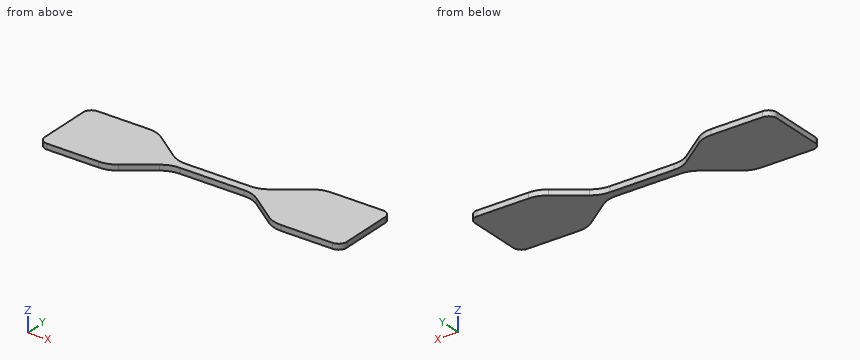
Autodesk Inventor part; units mm, degrees
ref_plane "YZ Plane" through (0, 0, 0) normal (1, 0, 0) x (0, 1, 0)
ref_plane "XZ Plane" through (0, 0, 0) normal (0, 1, 0) x (-1, 0, 0)
ref_plane "XY Plane" through (0, 0, 0) normal (0, 0, 1) x (1, 0, 0)
sketch "Sketch1" plane through (0, 0, 0) normal (0, 0, 1) x (1, 0, 0)
  line L0 (0, 0) -> (25, 0)
  line L1 (25, 25) -> (0, 25)
  line L2 (0, 25) -> (0, 0)
  line L3 (40, 14) -> (70, 14)
  line L4 (70, 11) -> (40, 11)
  line L5 (85, 0) -> (110, 0)
  line L6 (110, 0) -> (110, 25)
  line L7 (110, 25) -> (85, 25)
  line L8 (25, 25) -> (40, 14)
  line L9 (25, 0) -> (40, 11)
  line L10 (70, 14) -> (85, 25)
  line L11 (70, 11) -> (85, 0)
  point P0 (45, 12.5)
  point P1 (25, 12.5)
  dimension "d0" = 25
  dimension "d1" = 25
  dimension "d5" = 25
  dimension "d6" = 110
  dimension "d12" = 3
  dimension "d13" = 1.5
  dimension "d14" = 30
extrude "Extrusion1" add sketch "Sketch1" along normal blind 2
fillet "Fillet1" radius 10 8 edges at (25, 25, 1) (40, 14, 1) (70, 14, 1) (85, 25, 1) (25, 0, 1) (40, 11, 1) (70, 11, 1) (85, 0, 1)
fillet "Fillet2" radius 3 4 edges at (0, 25, 1) (0, 0, 1) (110, 25, 1) (110, 0, 1)
properties part number "Tensile Test Specimen"
CAD build for the part. Positions are in the model's coordinates, mm. Give positions to 0.01 mm unless a question says otherwise; leave off trailing zeros. Write each loop counter-clockwise with the first axis right and the second up, starting at its lowest first coordinate (ties: lowest second). Pieces come first, ordered by that corner, then holes. Notation, with made-up numbers: M 32,-17 L 42,-17 A6 cw 42,-11 Z; hole C 30.25,61 d1. An arc over 180 degrees is marked long. Return JSON: item names as keys, results as strings. Group by question number.
(1) Band-saw the part on C-C (x = 79). Give the cut face in (y, z), and give its area (3 significant figures).
(2) Flat gauge pins, fed straight in: pin 1 Ø0.6 at (x, z) = (57.5, 1.5) entering from -Y; pin 2 Ø3 at (x, y) = (75, 8.5) entering from -Z; pin 3 Ø0.6 at (x, z) = (56, 1.5) entering from +Y. Where does each tip first touch, or does it go through?
(3) Band-saw the part on B-B (y = 4.25). Give the cut face in (x, z).
(4) Band-saw the part on A-A (z = 1). Give the cut face in (x, y), and give its area (3 significant figures).
(5) Drill centre lines: L1, parallel to Y at x = 22, z = 0.8; L2, parallel to X at y = 18.25, z = 0.7; L3, parallel to X at y = 22.75, z = 0.45. Where is each one in solid material? Low to high. Write a range as [from, to].
(6) Band-saw the part on D-D (y = 10). Give the cut face in (x, z), and give its area (3 significant figures).
Entries:
{
 "1": {"outline": "M 4.4,0 L 20.6,0 L 20.6,2 L 4.4,2 Z", "area": "32.4 mm^2"},
 "2": {"pin 1": "stops at y = 11", "pin 2": "stops at z = 0", "pin 3": "stops at y = 14"},
 "3": {"outline": "M 0,0 L 30.8,0 L 30.8,2 L 0,2 Z; M 79.2,0 L 110,0 L 110,2 L 79.2,2 Z"},
 "4": {"outline": "M 0,3 A3 ccw 3,0 L 21.73,0 A10 ccw 27.64,1.94 L 37.36,9.06 A10 cw 43.27,11 L 66.73,11 A10 cw 72.64,9.06 L 82.36,1.94 A10 ccw 88.27,0 L 107,0 A3 ccw 110,3 L 110,22 A3 ccw 107,25 L 88.27,25 A10 ccw 82.36,23.06 L 72.64,15.94 A10 cw 66.73,14 L 43.27,14 A10 cw 37.36,15.94 L 27.64,23.06 A10 ccw 21.73,25 L 3,25 A3 ccw 0,22 Z", "area": "1,750 mm^2"},
 "5": {"L1": "y = [0, 25]", "L2": "x = [0, 34.2], [75.8, 110]", "L3": "x = [0.1, 28.07], [81.93, 109.9]"},
 "6": {"outline": "M 0,0 L 38.91,0 L 38.91,2 L 0,2 Z; M 71.09,0 L 110,0 L 110,2 L 71.09,2 Z", "area": "156 mm^2"}
}
